Work out the finished part from the listing and answer in its coordinate system (mm). A direction names the side the tool comes from. Give positions to 0.01 mm unless a question says otherwise; leave off trailing zeros. Loops run counter-clockwise (first coordinate to the right, second up) from the corner with the lowest first, then second, coordinate; pieces in that order, holes last. Notation, with made-up numbers: (-17.5, 57) -> (-1.5, 57) arc R7 ccw to (-1.5, 69) -> close; hole circle Ø3 at (78, -38). An arc over 180 degrees is marked (long way). Answer as CSV lines item,"result". Start each with the question number.
1. Find section C-C, the plane y = -101. Give the vertices of the cut face in (x, z).
2. Find the intervals of material crossed by line 1 along Z through (x, y) = (1.5, -510); line 2 along X through (y, z) = (-530, -0.25), in increasing order.
3. A tool of negligible diameter and unlimited length cuts with its end or side. For faces 4 (the face through (6.5, -625, -6.5)), 5 (the face through (3, -600, -10)), from which of +Z, -Z, +X, -X, +Y, -Y can it reach the whole face along a straight path? Write none if from no direction.
4. Find section B-B, the plane x = 0. Give the vertices of the cut face in (y, z), and give its area (3 significant figures).
5. Flat-ended cylindrical pins translate along their axes: pin 1 Ø4 at (x, y) = (10.5, -108) entering from +Z; pin 2 Ø1 at (x, y) = (4.5, -67.5) entering from -Z; pin 3 Ø1 at (y, z) = (-289, -11) entering from -X; pin 4 Ø10 at (x, y) = (6.5, -203.5) entering from +Z. Find the tip coordinate at first contact, or state that the pin passes through.
6. Determine the mould class of faces 1 (the face through (-9, 0, 2)), 2 (the face through (-2.17, -295.8, -9.76)), 3 (the face through (-1.172, -316.875, 8.923)) for opening direction Z: +Z half, -Z half, draft (parallel to the pull), parting line (faces both ways), or undercut.
7. Find section A-A, the plane z = 0. Give the vertices of the cut face in (x, y), and give its area (3 significant figures).
from build123d import *

# Parameters (mm, degrees)
F0_R     = 10
F1_DEPTH = 600
F2_R     = 15
F2_R_2   = 10
F3_DEPTH = 25
F4_R     = 9
F5_DEPTH = 700


with BuildPart() as f1:
    # F0 (on Front) → F1 (new body)
    with BuildSketch(Plane.XZ):
        Circle(F0_R)
    extrude(amount=F1_DEPTH)

    # F2 (on face) → F3 (join)
    with BuildSketch(Plane.XZ.offset(600)):
        Circle(F2_R)
        Circle(F2_R_2, mode=Mode.SUBTRACT)
        Circle(F2_R_2)
    extrude(amount=F3_DEPTH)

    # F4 (on face) → F5 (cut)
    with BuildSketch(Plane.XZ.offset(625)):
        Circle(F4_R)
    extrude(amount=-F5_DEPTH, mode=Mode.SUBTRACT)


solid = f1.part
Resolved:
1,outline,"circle Ø20 at (0, 0); hole circle Ø18 at (0, 0)"
2,line 1,"z = -9.89 to -8.87, 8.87 to 9.89"
2,line 2,"x = -10 to -9, 9 to 10"
3,face 4,"+Z, -Z, +X, -X, -Y"
3,face 5,"+Y"
4,outline,"(-625, -15) -> (-600, -15) -> (-600, -10) -> (0, -10) -> (0, -9) -> (-625, -9) -> close; (-625, 9) -> (0, 9) -> (0, 10) -> (-600, 10) -> (-600, 15) -> (-625, 15) -> close"
4,area,"1,500 mm^2"
5,pin 1,"stops at z = 5.27"
5,pin 2,"stops at z = -9.17"
5,pin 3,"passes through"
5,pin 4,"stops at z = 9.89"
6,face 1,"draft"
6,face 2,"parting line"
6,face 3,"undercut"
7,outline,"(-15, -625) -> (-9, -625) -> (-9, 0) -> (-10, 0) -> (-10, -600) -> (-15, -600) -> close; (9, -625) -> (15, -625) -> (15, -600) -> (10, -600) -> (10, 0) -> (9, 0) -> close"
7,area,"1,500 mm^2"
